Build history of the part. All positions in model axes, mm. Give positions to 0.01 mm unless a question says otherwise; leave off trailing zeros. Order: outer loops, then holes, each group sorted by start corner. A loop starts at its lowest first (then second) coordinate and runs counter-clockwise, first axis right, second up. Notation, with made-up numbers: (75, 85.25) -> (109, 85.25) arc R13 ccw to (109, 93.25) -> close; hole circle Ø8 at (89.25, -30.5). An arc over 180 degrees is marked (long way). One line per question, with ' | ' between items. Start each with the question number.
(1) Drill centre lines: L1, parallel to Y at x = 0, z = 2.9; L2, parallel to X at y = 23.5, z = 0.7; L3, parallel to Y at x = 15.5, z = 2.95. Where is each one in solid material? Low to high. Write a range as from..to.
(2) Pull direction X, two halves, no side cores. Call faces 1 (the face through (-17.2, -19.1, 0)), 2 (the face through (-21.62, 19.83, 1.89)), 3 (the face through (24.348, 7.668, 1.878)): +X half, -X half, draft (parallel to the pull), parting line (faces both ways), or undercut.
(3) Pin check, flat tips, straight feed: pin 1 Ø1.5 at (x, z) = (-14.5, 3.5) entering from +Y; pin 2 Ø1 at (y, z) = (4, 2) entering from +X; pin 3 Ø1.5 at (x, z) = (-7, 0.5) entering from -Y. Stop position of each tip, or through.
(4) Cut at A-A (x = 0). Give the cut face in (y, z), then the cut area to 3 significant figures.
(5) Cut at C-C (z = 2.5). Give the cut face in (x, y), then the cut area to 3 significant figures.
from build123d import *

# Parameters (mm, degrees)
F0_R     = 29.337
F0_R_2   = 25.527
F1_DEPTH = 3.81
F2_R     = 0.508
F3_R     = 0.508


with BuildPart() as f1:
    # F0 (on Top) → F1 (new body)
    with BuildSketch(Plane.XY):
        Circle(F0_R)
        Circle(F0_R_2, mode=Mode.SUBTRACT)
    extrude(amount=F1_DEPTH)

    # F2
    f2_edges = [f1.edges().sort_by_distance(p)[0] for p in [
        (-29.337, 0, 3.81),
    ]]
    fillet(f2_edges, radius=F2_R)

    # F3
    f3_edges = [f1.edges().sort_by_distance(p)[0] for p in [
        (-29.337, 0, 0),
    ]]
    fillet(f3_edges, radius=F3_R)


solid = f1.part
Result set:
1) L1: y = -29.34..-25.53, 25.53..29.34 | L2: x = -17.56..-9.97, 9.97..17.56 | L3: y = -24.91..-20.28, 20.28..24.91
2) face 1: draft | face 2: parting line | face 3: undercut
3) pin 1: stops at y = 25.9 | pin 2: stops at x = 29.13 | pin 3: stops at y = -28.66
4) outline: (-29.34, 0.51) arc R0.51 ccw to (-28.83, 0) -> (-25.53, 0) -> (-25.53, 3.81) -> (-28.83, 3.81) arc R0.51 ccw to (-29.34, 3.3) -> close; (25.53, 0) -> (28.83, 0) arc R0.51 ccw to (29.34, 0.51) -> (29.34, 3.3) arc R0.51 ccw to (28.83, 3.81) -> (25.53, 3.81) -> close | area: 28.8 mm2
5) outline: circle Ø58.67 at (0, 0); hole circle Ø51.05 at (0, 0) | area: 657 mm2
